Build history of the part. All positions in model axes, mm. A direction names the side the tool comes from. Coordinates: 2 decimals unless noted, no trailing zeros. Order: outer loops, then holes, each group sorted by start corner. A loop starts at its lowest first (then second) coordinate and runs counter-clockwise, first axis right, second up. Notation, with made-up numbers: (70.5, -23.75) - (114.5, -23.75) arc R27 cw to (114.5, 10.25) - close; hole circle Ø3 at (26, -23). An arc over 180 degrees is marked (long way). Write each question's results on one line, items separated by ' | '.
from build123d import *

# Parameters (mm, degrees)
SKETCH1_W           = 80
SKETCH1_H           = 60
BOSS_EXTRUDE1_DEPTH = 30
SKETCH2_W           = 37.144630664
SKETCH2_H           = 2.25
BOSS_EXTRUDE2_DEPTH = 22.5
SKETCH3_W           = 3
SKETCH3_H           = 24
BOSS_EXTRUDE3_DEPTH = 8.5
SKETCH5_R           = 1.575
CUT_EXTRUDE1_DEPTH  = 30
FILLET2_R           = 0.5


with BuildPart() as part:
    # Sketch1 → Boss-Extrude1 (new body)
    with BuildSketch(Plane.XY):
        with Locations((-96.427201848, 129.115774072)):
            Rectangle(SKETCH1_W, SKETCH1_H)
    extrude(amount=BOSS_EXTRUDE1_DEPTH)

    # Sketch2 → Boss-Extrude2 (add)
    with BuildSketch(Plane(origin=(0, 159.115774072, 0), x_dir=(1, 0, 0), z_dir=(0, 1, 0))):
        with Locations((-82.11807708, -3.375)):
            Rectangle(SKETCH2_W, SKETCH2_H)
        with Locations((-82.11807708, -26.625)):
            Rectangle(SKETCH2_W, SKETCH2_H)
    extrude(amount=BOSS_EXTRUDE2_DEPTH)

    # Sketch3 → Boss-Extrude3 (add)
    with BuildSketch(Plane(origin=(0, 159.115774072, 0), x_dir=(1, 0, 0), z_dir=(0, 1, 0))):
        with Locations((-128.777201848, -15)):
            Rectangle(SKETCH3_W, SKETCH3_H)
    extrude(amount=BOSS_EXTRUDE3_DEPTH)

    # Sketch5 → Cut-Extrude1 (cut)
    with BuildSketch(Plane(origin=(0, 0, 2.25), x_dir=(-1, 0, 0), z_dir=(0, 0, -1))):
        with Locations((95.090392412, 161.715774072)):
            Circle(SKETCH5_R)
        with Locations((95.090392412, 179.215774072)):
            Circle(SKETCH5_R)
    extrude(amount=-CUT_EXTRUDE1_DEPTH, mode=Mode.SUBTRACT)

    # Fillet2
    fillet2_edges = [part.edges().sort_by_distance(p)[0] for p in [
        (-56.427201848, 129.115774072, 30),
        (-100.690392412, 170.365774072, 2.25),
        (-100.690392412, 170.365774072, 4.5),
        (-96.427201848, 159.115774072, 30),
        (-63.545761748, 170.365774072, 4.5),
        (-63.545761748, 170.365774072, 2.25),
        (-100.690392412, 181.615774072, 3.375),
        (-82.11807708, 181.615774072, 4.5),
        (-63.545761748, 181.615774072, 3.375),
        (-82.11807708, 181.615774072, 2.25),
        (-100.690392412, 170.365774072, 25.5),
        (-100.690392412, 170.365774072, 27.75),
        (-63.545761748, 170.365774072, 27.75),
        (-63.545761748, 170.365774072, 25.5),
        (-100.690392412, 181.615774072, 26.625),
        (-82.11807708, 181.615774072, 27.75),
        (-63.545761748, 181.615774072, 26.625),
        (-82.11807708, 181.615774072, 25.5),
        (-130.277201848, 163.365774072, 3),
        (-130.277201848, 163.365774072, 27),
        (-127.277201848, 163.365774072, 27),
        (-127.277201848, 163.365774072, 3),
        (-130.277201848, 167.615774072, 15),
        (-127.277201848, 167.615774072, 15),
        (-136.427201848, 129.115774072, 30),
        (-96.427201848, 159.115774072, 0),
        (-56.427201848, 129.115774072, 0),
        (-136.427201848, 129.115774072, 0),
        (-136.427201848, 159.115774072, 15),
        (-56.427201848, 159.115774072, 15),
    ]]
    fillet(fillet2_edges, radius=FILLET2_R)


solid = part.part
1. Band-saw the part on A-A on y = 171.5. Give the cut face in (x, z), then the cut area to 3 significant figures.
Solved:
outline: (-100.69, 2.75) arc R0.5 ccw to (-100.19, 2.25) - (-64.05, 2.25) arc R0.5 ccw to (-63.55, 2.75) - (-63.55, 4) arc R0.5 ccw to (-64.05, 4.5) - (-100.19, 4.5) arc R0.5 ccw to (-100.69, 4) - close; (-100.69, 26) arc R0.5 ccw to (-100.19, 25.5) - (-64.05, 25.5) arc R0.5 ccw to (-63.55, 26) - (-63.55, 27.25) arc R0.5 ccw to (-64.05, 27.75) - (-100.19, 27.75) arc R0.5 ccw to (-100.69, 27.25) - close | area: 167 mm2
2. Probe line 1 (Y direction, x = -107, z = 15); line 2 (Z direction, x = -129, y = 166.5); line 3 (X direction, y = 173, z = 2.5). List the from-to ranges inside material, lowest first.
Solved:
line 1: y = 99.12 to 159.12 | line 2: z = 3 to 27 | line 3: x = -100.62 to -63.61
3. Band-saw the part on B-B on z = 12.5. Give the cut face in (x, y).
Solved:
outline: (-136.43, 99.12) - (-56.43, 99.12) - (-56.43, 158.62) arc R0.5 ccw to (-56.93, 159.12) - (-127.28, 159.12) - (-127.28, 167.12) arc R0.5 ccw to (-127.78, 167.62) - (-129.78, 167.62) arc R0.5 ccw to (-130.28, 167.12) - (-130.28, 159.12) - (-135.93, 159.12) arc R0.5 ccw to (-136.43, 158.62) - close
4. Drop flat-ended pins along their axis: pin 1 Ø2.5 at (y, z) = (165, 14.5) entering from -X; pin 2 Ø5 at (x, z) = (-112, 10.5) entering from +Y; pin 3 Ø2 at (x, y) = (-128.5, 162.5) entering from -Z. Give the stop position or say it passes through.
Solved:
pin 1: stops at x = -130.28 | pin 2: stops at y = 159.12 | pin 3: stops at z = 3
5. Band-saw the part on C-C on x = -107.5. Give the cut face in (y, z).
Solved:
outline: (99.12, 0) - (158.62, 0) arc R0.5 ccw to (159.12, 0.5) - (159.12, 29.5) arc R0.5 ccw to (158.62, 30) - (99.12, 30) - close
6. Tool access for faces 4 (the face through (-82, 170, 4.5)), 5 (the face through (-82, 170, 2.25)), 6 (the face through (-129, 163, 27)): list every direction of +Z, -Z, +X, -X, +Y, -Y with a clear straight run to the whole face (end or side of a thin tool).
Solved:
face 4: +X, +Y | face 5: -Z, +X, -X, +Y | face 6: +Z, -X, +Y
7. Two-plate mould, pull along X, no slides. Class faces 1 (the face through (-95.82, 177.82, 26.61)), 2 (the face through (-56.427, 128, 15)), 3 (the face through (-82, 170, 27.75)): +X half, -X half, draft (parallel to the pull), parting line (faces both ways), or undercut.
Solved:
face 1: undercut | face 2: +X half | face 3: draft
